from build123d import *

# Parameters (mm, degrees)
SKETCH1_R           = 20
BOSS_EXTRUDE1_DEPTH = 25
CUT_EXTRUDE1_REACH  = 22
SKETCH2_W           = 45.354369025
SKETCH2_H           = 3.724754944
SKETCH2_H_2         = 2.877438925
SKETCH2_H_3         = 3.230053013
CUT_EXTRUDE2_REACH  = 22
SKETCH3_W           = 39.909801602
SKETCH3_H           = 0.954143847
SKETCH4_R           = 3
CUT_EXTRUDE3_DEPTH  = 51
SKETCH5_R           = 4
CUT_EXTRUDE4_DEPTH  = 10


with BuildPart() as part:
    # Sketch1 → Boss-Extrude1 (new body, symmetric)
    with BuildSketch(Plane.XY):
        Circle(SKETCH1_R)
    extrude(amount=BOSS_EXTRUDE1_DEPTH, both=True)

    # Sketch2 → Cut-Extrude1 (cut, up to next)
    with BuildSketch(Plane(origin=(0, 0, 0), x_dir=(1, 0, 0), z_dir=(0, 1, 0)), mode=Mode.PRIVATE) as cut_extrude1_sk1:
        with Locations((0.618163083, 17.131545904)):
            Rectangle(SKETCH2_W, SKETCH2_H)
    cut_extrude1_tool1 = extrude(cut_extrude1_sk1.sketch, amount=-CUT_EXTRUDE1_REACH, mode=Mode.PRIVATE) & part.part
    add(cut_extrude1_tool1.solids().sort_by_distance((0.618163, 0, -17.131546))[0], mode=Mode.SUBTRACT)
    # Sketch2 → Cut-Extrude1 (cut, up to next)
    with BuildSketch(Plane(origin=(0, 0, 0), x_dir=(1, 0, 0), z_dir=(0, 1, 0)), mode=Mode.PRIVATE) as cut_extrude1_sk2:
        with Locations((0.618163083, 2.232701411)):
            Rectangle(SKETCH2_W, SKETCH2_H_2)
    cut_extrude1_tool2 = extrude(cut_extrude1_sk2.sketch, amount=-CUT_EXTRUDE1_REACH, mode=Mode.PRIVATE) & part.part
    add(cut_extrude1_tool2.solids().sort_by_distance((0.618163, 0, -2.232701))[0], mode=Mode.SUBTRACT)
    # Sketch2 → Cut-Extrude1 (cut, up to next)
    with BuildSketch(Plane(origin=(0, 0, 0), x_dir=(1, 0, 0), z_dir=(0, 1, 0)), mode=Mode.PRIVATE) as cut_extrude1_sk3:
        with Locations((0.618163083, -8.81108963)):
            Rectangle(SKETCH2_W, SKETCH2_H_3)
    cut_extrude1_tool3 = extrude(cut_extrude1_sk3.sketch, amount=-CUT_EXTRUDE1_REACH, mode=Mode.PRIVATE) & part.part
    add(cut_extrude1_tool3.solids().sort_by_distance((0.618163, 0, 8.81109))[0], mode=Mode.SUBTRACT)

    # Sketch3 → Cut-Extrude2 (cut, up to next)
    with BuildSketch(Plane(origin=(0, 0, 0), x_dir=(1, 0, 0), z_dir=(0, 1, 0)), mode=Mode.PRIVATE) as cut_extrude2_sk1:
        with Locations((-0.045099199, -0.477071924)):
            Rectangle(SKETCH3_W, SKETCH3_H)
    cut_extrude2_tool1 = extrude(cut_extrude2_sk1.sketch, amount=CUT_EXTRUDE2_REACH, mode=Mode.PRIVATE) & part.part
    add(cut_extrude2_tool1.solids().sort_by_distance((-0.045099, 0, 0.477072))[0], mode=Mode.SUBTRACT)

    # Sketch4 → Cut-Extrude3 (cut, through all)
    with BuildSketch(Plane(origin=(0, 0, -25), x_dir=(-1, 0, 0), z_dir=(0, 0, -1))):
        Circle(SKETCH4_R)
    extrude(amount=-CUT_EXTRUDE3_DEPTH, mode=Mode.SUBTRACT)

    # Sketch5 → Cut-Extrude4 (cut)
    with BuildSketch(Plane(origin=(0, 0, -25), x_dir=(-1, 0, 0), z_dir=(0, 0, -1))):
        Circle(SKETCH5_R)
    extrude(amount=-CUT_EXTRUDE4_DEPTH, mode=Mode.SUBTRACT)


solid = part.part
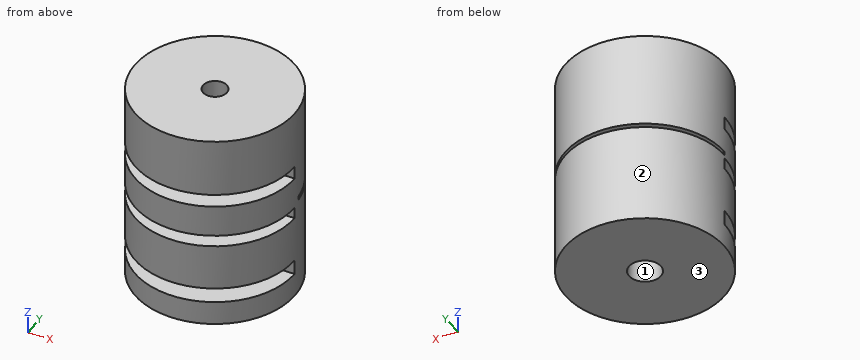
The model under review builds one solid part; all positions refer to its coordinate system, in mm. Face numbers are marked on the shaded views. Round coordinates to 2 decimals unless told otherwise and drop trailing zeros. Write each loop counter-clockwise with the first axis right and the second up, starting at its lowest first coordinate (ties: lowest second). Pieces come first, ordered by that corner, then holes. Notation, with made-up numbers: M 56.5,13.5 L 92.5,13.5 A14 ccw 92.5,38.5 Z; hole C 51,25 d8. An arc over 180 degrees is marked long. Answer as CSV lines item,"result". Start each with the question number.
Q1. Wall thickness on line 1 along Z through (x, y) = (15, -2); line 2 along Z through (x, y) = (0.5, 8.5); line 3 along Y through (x, z) = (0, 12): over which ranges is each line inside the solid? List them lowest first.
Q2. Consider section C-C, the plane y = 17. Give the boundary of the cut face in (x, z).
Q3. Consider section B-B, the plane x = 0. Give the boundary of the cut face in (y, z).
Q4. The part is to be moulded in two halves that separate along Y. For the marked faces 1, 2 and 3, say which applies: +Y half, -Y half, draft (parallel to the pull), parting line (faces both ways), or undercut.
Q5. Consider section D-D, the plane x = 16.5. Give the boundary of the cut face in (y, z), then the cut area to 3 significant figures.
Q6. Consider section A-A, the plane y = -6. Give the boundary of the cut face in (x, z), then the cut area to 3 significant figures.
Q7. Clearance check with flat-ended pins moving along their axes: P1, Ø3, axis at x = -13.5, z = -17, coming from the -Y side; P2, Ø5, axis at y = -10.5, z = -3, coming from the -X side; P3, Ø5, axis at x = 0, y = 0, coming from the +Z side; P4, Ø5, axis at x = -8, z = 17.5, coming from the +Y side. State where each tip first meets the part, or that it passes through.
Result set:
1,line 1,"z = -25 to -18.99, -15.27 to -3.67, -0.79 to 7.2, 10.43 to 25"
1,line 2,"z = -25 to 0, 0.95 to 25"
1,line 3,"y = -20 to -3, 3 to 20"
2,outline,"M -10.54,-25 L 10.54,-25 L 10.54,0 L -10.54,0 Z; M -10.54,0.95 L 10.54,0.95 L 10.54,25 L -10.54,25 Z"
3,outline,"M -20,-25 L -4,-25 L -4,-18.99 L -20,-18.99 Z; M -20,-15.27 L -4,-15.27 L -4,-15 L -3,-15 L -3,-3.67 L -20,-3.67 Z; M -20,-0.79 L -3,-0.79 L -3,7.2 L -20,7.2 Z; M -20,10.43 L -3,10.43 L -3,25 L -20,25 Z; M 3,-15 L 4,-15 L 4,-25 L 20,-25 L 20,0 L 3,0 Z; M 3,0.95 L 20,0.95 L 20,25 L 3,25 Z"
4,face 1,"undercut"
4,face 2,"parting line"
4,face 3,"draft"
5,outline,"M -11.3,-25 L 11.3,-25 L 11.3,0 L 0,0 L 0,0.95 L 11.3,0.95 L 11.3,25 L -11.3,25 L -11.3,10.43 L 0,10.43 L 0,7.2 L -11.3,7.2 L -11.3,-0.79 L 0,-0.79 L 0,-3.67 L -11.3,-3.67 L -11.3,-15.27 L 0,-15.27 L 0,-18.99 L -11.3,-18.99 Z"
5,area,"1,010 mm²"
6,outline,"M -19.08,-25 L 19.08,-25 L 19.08,-18.99 L -19.08,-18.99 Z; M -19.08,-15.27 L 19.08,-15.27 L 19.08,-3.67 L -19.08,-3.67 Z; M -19.08,-0.79 L 19.08,-0.79 L 19.08,7.2 L -19.08,7.2 Z; M -19.08,10.43 L 19.08,10.43 L 19.08,25 L -19.08,25 Z"
6,area,"1,530 mm²"
7,P1,"stops at y = 0"
7,P2,"stops at x = -18.29"
7,P3,"passes through"
7,P4,"stops at y = 19.23"
